from build123d import *

# Parameters (mm, degrees)
F0_W     = 150
F0_H     = 100
F1_DEPTH = 30
F2_R     = 3
F3_DEPTH = 5
F2_W     = 30.162632
F2_H     = 22.921
F4_DEPTH = 30
F5_W     = 20
F5_H     = 20
F6_DEPTH = 15
F7_R     = 4
F8_DEPTH = 40


with BuildPart() as f1:
    # F0 (on Top) → F1 (new body)
    with BuildSketch(Plane.XY):
        Rectangle(F0_W, F0_H)
    extrude(amount=F1_DEPTH)

    # F2 (on face) → F3 (join)
    with BuildSketch(Plane.XY.offset(30)):
        with Locations((-52.058708, -22.7105)):
            Circle(F2_R)
        with Locations((-52.058708, 22.7105)):
            Circle(F2_R)
    extrude(amount=F3_DEPTH)

    # F2 (on face) → F4 (join)
    with BuildSketch(Plane.XY.offset(30)):
        with Locations((-52.058708, 22.7105)):
            Rectangle(F2_W, F2_H)
        with Locations((-52.058708, 22.7105)):
            Circle(F2_R, mode=Mode.SUBTRACT)
        with Locations((-52.058708, -22.7105)):
            Rectangle(F2_W, F2_H)
        with Locations((-52.058708, -22.7105)):
            Circle(F2_R, mode=Mode.SUBTRACT)
    extrude(amount=F4_DEPTH)

    # F5 (on face) → F6 (join)
    with BuildSketch(Plane(origin=(0, 34.171, 0), x_dir=(-1, 0, 0), z_dir=(0, 1, 0))):
        with Locations((26.977392, 40)):
            Rectangle(F5_W, F5_H)
    extrude(amount=-F6_DEPTH)

    # F7 (on face) → F8 (join)
    with BuildSketch(Plane.XZ.offset(-19.171)):
        with Locations((-26.977392, 40)):
            Circle(F7_R)
    extrude(amount=F8_DEPTH)


solid = f1.part
Build history of the part. All positions in model axes, mm. A direction names the side the tool comes from. Coordinates: 2 decimals unless noted, no trailing zeros. Order: outer loops, then holes, each group sorted by start corner. A loop starts at its lowest first (then second) coordinate and runs counter-clockwise, first axis right, second up. Notation, with made-up numbers: (-17, 39) - (12, 39) arc R28 cw to (12, 66) - close; hole circle Ø3 at (56.25, -25). An arc over 180 degrees is marked (long way). Write item = value, one per line. Start each with the question number.
1) Saw through at C-C on x = -61. Write the cut outline in (y, z), then the cut area to 3 significant figures.
2) 3-axis set-ups, long thin cutter, end or side, ignore diameter. For faces 4 (the face through (-27, -20.829, 40)), 5 (the face through (-22, 19.171, 40)), 6 (the face through (-52, -23, 35)), 7 (the face through (-52, -34.171, 45)): which of +Z, -Z, +X, -X, +Y, -Y reach the whole face in a straight line?
3) Saw through at A-A on z = 48. Write the cut outline in (x, y).
4) Saw through at B-B on y = -4. Write the cut outline in (x, z).
5) Saw through at D-D on y = 42. Write the cut outline in (x, z).
6) Flat gauge pins, fed straight in: pin 1 Ø5.5 at (x, y) = (-52.06, 22.71) entering from +Z; pin 2 Ø6 at (x, y) = (17, -36) entering from +Z; pin 3 Ø10 at (y, z) = (10.5, 44) entering from +X. Where does each tip first touch, or does it go through?
7) Wall check: line 1 along Y through (x, z) = (-58, 46.5); line 2 along Z through (x, y) = (-8, -38.5); line 3 along Z through (x, y) = (-22.5, 31). Give the ranges that are in metal, low to high. Write a range as from..to.
8) Two-plate mould, pull along X, no slides. Class faces 1 (the face through (-56, 23, 60)), 2 (the face through (-67.14, -23, 45)), 3 (the face through (-36.977, 17, 48)): pulls with the +X half, pulls with the -X half, needs draft (parallel to the pull), parting line crosses it, or undercut.
From the geometry:
q1.outline = (-50, 0) - (50, 0) - (50, 30) - (34.17, 30) - (34.17, 60) - (11.25, 60) - (11.25, 30) - (-11.25, 30) - (-11.25, 60) - (-34.17, 60) - (-34.17, 30) - (-50, 30) - close
q1.area = 4,380 mm^2
q2.face_4 = +Z, +X, -Y
q2.face_5 = -Y
q2.face_6 = +Z
q2.face_7 = +Z, +X, -X, -Y
q3.outline = (-67.14, -34.17) - (-36.98, -34.17) - (-36.98, -11.25) - (-67.14, -11.25) - close; (-67.14, 11.25) - (-36.98, 11.25) - (-36.98, 19.17) - (-16.98, 19.17) - (-16.98, 34.17) - (-67.14, 34.17) - close; hole circle Ø6 at (-52.06, -22.71); hole circle Ø6 at (-52.06, 22.71)
q4.outline = (-75, 0) - (75, 0) - (75, 30) - (-75, 30) - close; circle Ø8 at (-26.98, 40)
q5.outline = (-75, 0) - (75, 0) - (75, 30) - (-75, 30) - close
q6.pin_1 = 35
q6.pin_2 = 30
q6.pin_3 = -22.98
q7.line_1 = -34.17..-11.25, 11.25..34.17
q7.line_2 = 0..30
q7.line_3 = 0..50
q8.face_1 = needs draft
q8.face_2 = pulls with the -X half
q8.face_3 = undercut
